Source: CAD feature listing. Evaluate the final solid. Frame: model axes, mm. Coordinates: 2 decimals unless noted, no trailing zeros. Loops run counter-clockwise (first coordinate to the right, second up) from the corner with the lowest first, then second, coordinate; pieces in that order, holes last.
from build123d import *

# Parameters (mm, degrees)
F0_W     = 508
F0_H     = 508
F1_DEPTH = 254
F3_DEPTH = 508.001
F5_DEPTH = 508


with BuildPart() as f1:
    # F0 (on Front) → F1 (new body)
    with BuildSketch(Plane.XZ):
        with Locations((254, 254)):
            Rectangle(F0_W, F0_H)
    extrude(amount=F1_DEPTH)

    # F2 (on face) → F3 (cut, through all)
    with BuildSketch(Plane.YZ.offset(508)):
        Polygon((-254, 508), (-254, 393.7), (0, 508), align=None)
        Polygon((0, 0), (-254, 114.3), (-254, 0), align=None)
    extrude(amount=-F3_DEPTH, mode=Mode.SUBTRACT)

    # F4 (on Top) → F5 (cut)
    with BuildSketch(Plane.XY):
        Polygon((0, -254), (114.3, -254), (0, 0), align=None)
        Polygon((393.7, -254), (508, -254), (542.023063, -254), (542.023063, 0), (508, 0), align=None)
    extrude(amount=F5_DEPTH, mode=Mode.SUBTRACT)


solid = f1.part
Q1. Section B-B, the plane y = -70. Return the cut outline in (x, z), plus the area to 3 significant figures.
Q2. Line query: line 1 along X through (y, z) = (-57, 327.5); line 2 along Y through (x, z) = (80.5, 285); line 3 along X through (y, z) = (-35, 258). Output: solid intervals per line, ascending.
Q3. Section A-A, the plane z = 146.5. Return the cut outline in (x, y), plus the area to 4 significant figures.
Q4. Contact query for flat-ended pins moving along their axis: pin 1 Ø2 at (x, z) = (168, 303.5) entering from +Y; pin 2 Ø4 at (y, z) = (-123.5, 377.5) entering from -X (3 decimals); pin 3 Ø2 at (x, y) = (456.5, -55.5) entering from -Z (3 decimals); pin 4 Ø1 at (x, y) = (196, -33) entering from -Z (3 decimals). Output: stop coordinate, or through.
Derived:
1. outline: (31.5, 31.5) - (476.5, 31.5) - (476.5, 476.5) - (31.5, 476.5) - close
1. area: 198,000 mm2
2. line 1: x = 25.65 to 482.35
2. line 2: y = -178.89 to 0
2. line 3: x = 15.75 to 492.25
3. outline: (0, 0) - (114.3, -254) - (393.7, -254) - (508, 0) - close
3. area: 100,000 mm2
4. pin 1: stops at y = 0
4. pin 2: stops at x = 54.675
4. pin 3: stops at z = 24.525
4. pin 4: stops at z = 14.625
